```python
from build123d import *

# Parameters (mm, degrees)
F0_R     = 1.5875
F0_R_2   = 1.5
F1_DEPTH = 3.175


with BuildPart() as f1:
    # F0 (on Front) → F1 (new body)
    with BuildSketch(Plane.XZ):
        with BuildLine():
            ThreePointArc((-12.7, 0), (0, -12.7), (12.7, 0))
            ThreePointArc((12.7, 0), (0, 12.7), (-12.7, 0))
        make_face()
        Circle(F0_R, mode=Mode.SUBTRACT)
        with BuildLine():
            ThreePointArc((-12.7, 0), (0, 12.7), (12.7, 0))
            Line((12.7, 0), (30.943444, 10.093794))
            ThreePointArc((30.943444, 10.093794), (50.110639, 28.743667), (57.15, 54.543794))
            ThreePointArc((57.15, 54.543794), (43.726088, 89.639294), (57.15, 124.734794))
            Line((57.15, 124.734794), (57.15, 145.243444))
            ThreePointArc((57.15, 145.243444), (53.430256, 154.2237), (44.45, 157.943444))
            Line((44.45, 157.943444), (-44.45, 157.943444))
            ThreePointArc((-44.45, 157.943444), (-53.430256, 154.2237), (-57.15, 145.243444))
            Line((-57.15, 145.243444), (-57.15, 124.734794))
            ThreePointArc((-57.15, 124.734794), (-43.726088, 89.639294), (-57.15, 54.543794))
            ThreePointArc((-57.15, 54.543794), (-50.110639, 28.743667), (-30.943444, 10.093794))
            Line((-30.943444, 10.093794), (-12.7, 0))
        make_face()
        with Locations((-25.4, 29.143794)):
            Circle(F0_R_2, mode=Mode.SUBTRACT)
        with Locations((0, 25.4)):
            Circle(F0_R, mode=Mode.SUBTRACT)
        with Locations((25.4, 29.143794)):
            Circle(F0_R_2, mode=Mode.SUBTRACT)
        with Locations((0, 63.5)):
            Circle(F0_R, mode=Mode.SUBTRACT)
        with Locations((-31.75, 79.943794)):
            Circle(F0_R_2, mode=Mode.SUBTRACT)
        with Locations((-44.45, 137.434794)):
            Circle(F0_R, mode=Mode.SUBTRACT)
        with Locations((-7.550921, 141.723698)):
            Circle(F0_R, mode=Mode.SUBTRACT)
        with Locations((0, 107.95)):
            Circle(F0_R, mode=Mode.SUBTRACT)
        with Locations((31.75, 79.943794)):
            Circle(F0_R_2, mode=Mode.SUBTRACT)
        with Locations((7.550921, 141.723698)):
            Circle(F0_R, mode=Mode.SUBTRACT)
        with Locations((44.45, 137.434794)):
            Circle(F0_R, mode=Mode.SUBTRACT)
    extrude(amount=F1_DEPTH)


solid = f1.part
```
Read the model definition and answer for the solid it produces. Units are mm, in the model's axes. Round coordinates to 2 decimals unless told otherwise and drop trailing zeros. Write each loop counter-clockwise with the first axis right and the second up, starting at its lowest first coordinate (ties: lowest second). Pieces come first, ordered by that corner, then holes. Notation, with made-up numbers: (-15.5, 14) -> (35.5, 14) arc R23 cw to (35.5, 31) -> close; hole circle Ø8 at (69.5, 80.25). An arc over 180 degrees is marked (long way). Answer in a Markdown table with one row per item. Add a question column.
1) Determine the mould class of faces 1 (the face through (7.207, -1.565, 140.174)), 2 (the face through (42.864, -1.565, 137.505)), 3 (the face through (43.73, -1.57, 89.1)), 4 (the face through (-50.3, -1.57, 29.07)) for opening direction X: pulls with the +X half, pulls with the -X half, needs draft (parallel to the pull), parting line crosses it, or undercut.
2) Find section C-C, the plane z = 87. Determine the outline of the cut face in (x, y) (3 decimals).
3) Find section B-B, the plane x = -22. Determine the outline of the cut face in (y, z) (3 decimals).
4) Find section A-A, the plane y = -2.1. State how many separate pieces and enclosed holes the cut face has, and give its area (3 significant figures).
5) Consider line 1 (Z direction, x = 0, y = -1); line 2 (X direction, y = -1.4, z = 138); line 3 (Z direction, x = -9, y = -1.15). Determine where each line is inside the solid, lowest interval first.
6) Given P1, Ø1, axis at x = 6.5, y = -2, coming from the -Z side; P2, Ø1, axis at y = -1.5, z = 106, coming from the +X side, each flat-ended and moving along its own axis, determine where each tip first touches the part or whether it passes through.
Findings below:
| question | item | result |
|---|---|---|
| 1 | face 1 | undercut |
| 1 | face 2 | undercut |
| 1 | face 3 | pulls with the +X half |
| 1 | face 4 | pulls with the -X half |
| 2 | outline | (-43.792, -3.175) -> (43.792, -3.175) -> (43.792, 0) -> (-43.792, 0) -> close |
| 3 | outline | (-3.175, 5.146) -> (0, 5.146) -> (0, 157.943) -> (-3.175, 157.943) -> close |
| 4 | separate pieces | 1 |
| 4 | enclosed holes | 12 |
| 4 | area | 15,500 mm² |
| 5 | line 1 | -12.7 to -1.59, 1.59 to 23.81, 26.99 to 61.91, 65.09 to 106.36, 109.54 to 157.94 |
| 5 | line 2 | -57.15 to -45.93, -42.97 to 42.97, 45.93 to 57.15 |
| 5 | line 3 | -8.96 to 141.08, 142.37 to 157.94 |
| 6 | P1 | z = -11.19 |
| 6 | P2 | x = 46.5 |
